Design review of the part built by this model. Coordinates are the model's own, in mm. Face numbers are marked on the shaded views. A direction names the side the tool comes from. Give positions to 0.01 mm unless a question says otherwise; leave off trailing zeros. Loops run counter-clockwise (first coordinate to the right, second up) from the corner with the lowest first, then second, coordinate; pieces in that order, holes last. Notation, with made-up numbers: M 57.25,36 L 116.25,36 A29 cw 116.25,70 Z; hole C -13,82 d8. An arc over 180 degrees is marked long. Use a Markdown table: item, result. Add a question column.
(1) Add section D-D, the plane z = 7.5. Give the boundary of the cut face in (x, y).
(2) Draft analysis for pull direction X (two halves, no side actions). For the marked faces 1, 2 and 3, state which applies: pulls with the +X half, pulls with the -X half, needs draft (parallel to the pull), parting line crosses it, or undercut.
(3) Add section C-C, the plane x = 1. Give the boundary of the cut face in (y, z), then the cut area to 3 significant figures.
(4) Add section A-A, the plane z = 28. Give the boundary of the cut face in (x, y), then the cut area to 4 significant figures.
(5) Add section B-B, the plane x = 13. Give the boundary of the cut face in (y, z).
(6) Insertion check: pin 1 Ø1.5 at (x, y) = (11.5, -68.5) entering from +Z; pin 2 Ø3 at (y, z) = (-62, 27.5) entering from +X; pin 3 Ø3 at (x, z) = (-36.5, 15.5) entering from -Y. Each pin has a flat end and moves straight along its axis. Give the tip position at first contact, or say it passes through.
(7) For the marked faces 4, 5 and 6, list the 3-axis set-ups (+Z, -Z, +X, -X, +Y, -Y) from which the entire face can be reached by the end or side of a thin tool; tool diameter is ignored.
(8) For probe 1 along Z at (x, y) = (5, -61.25); probe 2 along Y at (x, z) = (-32, 7); probe 3 along X at (y, z) = (-64.75, 24), list the stretches that pass through material, from the lowest coordinate up.
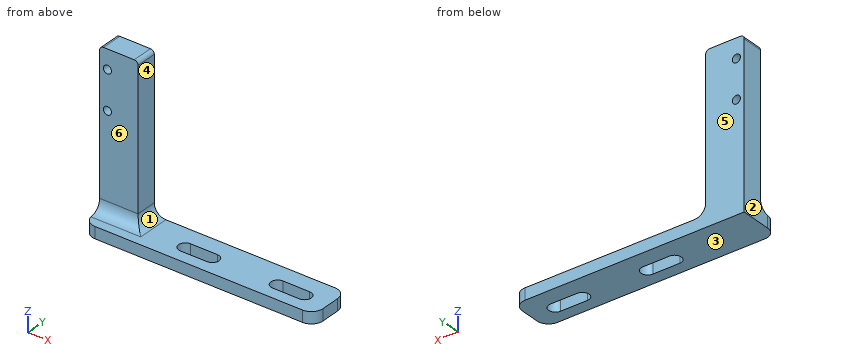
Autodesk Inventor part; units mm, degrees
ref_plane "YZ Plane" through (0, 0, 0) normal (1, 0, 0) x (0, 1, 0)
ref_plane "XZ Plane" through (0, 0, 0) normal (0, 1, 0) x (-1, 0, 0)
ref_plane "XY Plane" through (0, 0, 0) normal (0, 0, 1) x (1, 0, 0)
ref_plane "Work Plane1" through (0, 0, 0) normal (0, 0, 1) x (1, 0, 0)
sketch "Sketch1" plane through (0, 0, 0) normal (0, 0, 1) x (1, 0, 0)
  line L0 (18.2061, -59.3733) -> (-41.7939, -59.3733)
  line L1 (-41.7939, -59.3733) -> (-41.7939, -70.3733)
  line L2 (-41.7939, -70.3733) -> (18.2061, -70.3733)
  line L3 (18.2061, -70.3733) -> (18.2061, -59.3733)
  circle A0 centre (12, -65.5261) radius 1.75
  circle A1 centre (-12, -65.5261) radius 1.75
  line L4 (-12, -67.2761) -> (-12, -63.7761)
  line L5 (-12, -63.7761) -> (-19, -63.7761)
  line L6 (-19, -63.7761) -> (-19, -67.2761)
  line L7 (-19, -67.2761) -> (-12, -67.2761)
  line L8 (-12, -67.2761) -> (-12, -63.7761)
  line L9 (12, -67.2761) -> (12, -63.7761)
  line L10 (12, -63.7761) -> (5, -63.7761)
  line L11 (5, -63.7761) -> (5, -67.2761)
  line L12 (5, -67.2761) -> (12, -67.2761)
  line L13 (12, -67.2761) -> (12, -63.7761)
  circle A2 centre (-19, -65.5261) radius 1.75
  circle A3 centre (5, -65.5261) radius 1.75
  point P0 (0, 0)
  dimension "d0" = 60
  dimension "d1" = 11
  dimension "d13" = 7
  dimension "d14" = 7
extrude "Extrusion1" add sketch "Sketch1" along normal blind 3
sketch "Sketch2" plane through (0, 0, 3) normal (0, 0, 1) x (1, 0, 0)
  line L0 (-41.7939, -59.3733) -> (-41.7939, -70.3733)
  line L1 (-41.7939, -59.3733) -> (-31.7939, -59.3733)
  line L2 (-31.7939, -59.3733) -> (-31.7939, -64.8733)
  line L3 (-31.7939, -64.8733) -> (-41.7939, -64.8733)
  line L4 (-41.7939, -64.8733) -> (-41.7939, -59.3733)
  point P0 (0, 0)
  dimension "d4" = 10
  dimension "d5" = 5.5
extrude "Extrusion2" add sketch "Sketch2" along normal blind 40
sketch "Sketch3" plane through (-41.7939, -64.8733, 3) normal (0, -1, 0) x (1, 0, 0)
  circle A0 centre (2.0172, 35) radius 1.05
  circle A1 centre (2.0172, 25) radius 1.05
  point P0 (41.7939, -3)
extrude "Extrusion3" cut sketch "Sketch3" against normal blind 5.5
fillet "Fillet1" radius 1 2 edges at (-41.7939, -62.1233, 43) (-31.7939, -62.1233, 43)
fillet "Fillet2" radius 3 2 edges at (-36.7939, -64.8733, 3) (-31.7939, -62.1233, 3)
fillet "Fillet3" radius 3 3 edges at (18.2061, -59.3733, 1.5) (18.2061, -70.3733, 1.5) (-41.7939, -70.3733, 1.5)
properties part number "Homing_switch_holder"
Established:
| question | item | result |
|---|---|---|
| 1 | outline | M -41.79,-64.87 L -31.79,-64.87 L -31.79,-59.37 L -41.79,-59.37 Z |
| 2 | face 1 | pulls with the +X half |
| 2 | face 2 | pulls with the -X half |
| 2 | face 3 | needs draft |
| 3 | outline | M -70.37,0 L -59.37,0 L -59.37,3 L -70.37,3 Z |
| 3 | area | 33.0 mm^2 |
| 4 | outline | M -41.79,-64.87 L -40.83,-64.87 L -40.83,-59.37 L -41.79,-59.37 Z; M -38.73,-64.87 L -31.79,-64.87 L -31.79,-59.37 L -38.73,-59.37 Z |
| 4 | area | 43.45 mm^2 |
| 5 | outline | M -70.37,0 L -66.96,0 L -66.96,3 L -70.37,3 Z; M -64.09,0 L -59.37,0 L -59.37,3 L -64.09,3 Z |
| 6 | pin 1 | z = 3 |
| 6 | pin 2 | x = -31.79 |
| 6 | pin 3 | y = -64.87 |
| 7 | face 4 | +Z, +X, +Y, -Y |
| 7 | face 5 | +Z, -Z, +X, -X, +Y |
| 7 | face 6 | +Z, +X, -X, -Y |
| 8 | probe 1 | 0 to 3 |
| 8 | probe 2 | -64.87 to -59.37 |
| 8 | probe 3 | -41.79 to -31.79 |
